Geometry: see drawing. Coordinates: mm, zero at the bounding-box minimum. Coordinates: 2 decimals unless noted, no trailing zeros. Write each loop counter-clockwise with the first axis right and the second up, starting at its lowest first coordinate (ties: lowest second). Pieces come first, ordered by that corner, then holes. Notation, with made-up numbers: M 66,-8 L 107,-8 A33 cw 107,22 Z; hole C 5,-15 d8. An arc over 180 degrees is marked long. Answer as CSV lines item,"result". Start each with the question number.
1. Section C-C on z = 9. Return the cut outline in (x, y), plus the area to 3 significant figures.
2. Line query: probe 1 along X at (y, z) = (0.4, 10.5); probe 2 along Z at (x, y) = (104, 3.3); probe 3 along Z at (x, y) = (87.5, 0.25). Output: solid intervals per line, ascending. Write a range as [from, to].
3. Contact query for flat-ended pins moving along their axis: pin 1 Ø2.5 at (y, z) = (2.5, 13.5) entering from -X; pin 2 Ø1.5 at (y, z) = (1.5, 18.5) entering from +X. Output: stop coordinate, or through.
4. Section A-A on y = 2.5. Return the cut outline in (x, z).
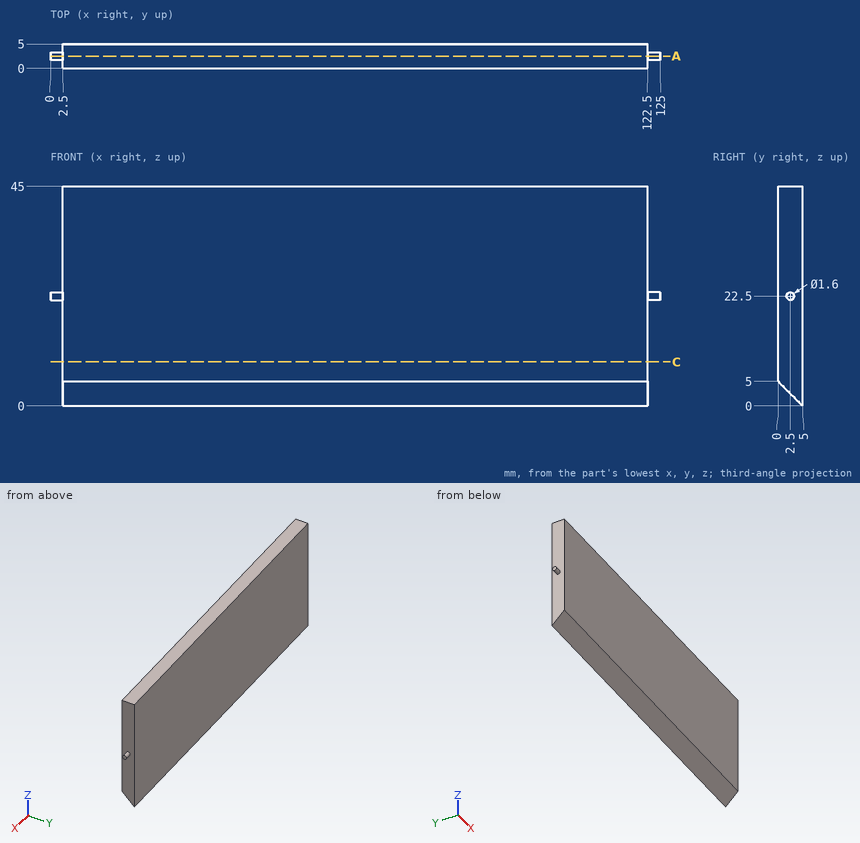
Values:
1,outline,"M 2.5,0 L 122.5,0 L 122.5,5 L 2.5,5 Z"
1,area,"600 mm²"
2,probe 1,"[2.5, 122.5]"
2,probe 2,"[1.7, 45]"
2,probe 3,"[4.75, 45]"
3,pin 1,"x = 2.5"
3,pin 2,"x = 122.5"
4,outline,"M 0,21.7 L 2.5,21.7 L 2.5,2.5 L 122.5,2.5 L 122.5,21.7 L 125,21.7 L 125,23.3 L 122.5,23.3 L 122.5,45 L 2.5,45 L 2.5,23.3 L 0,23.3 Z"
